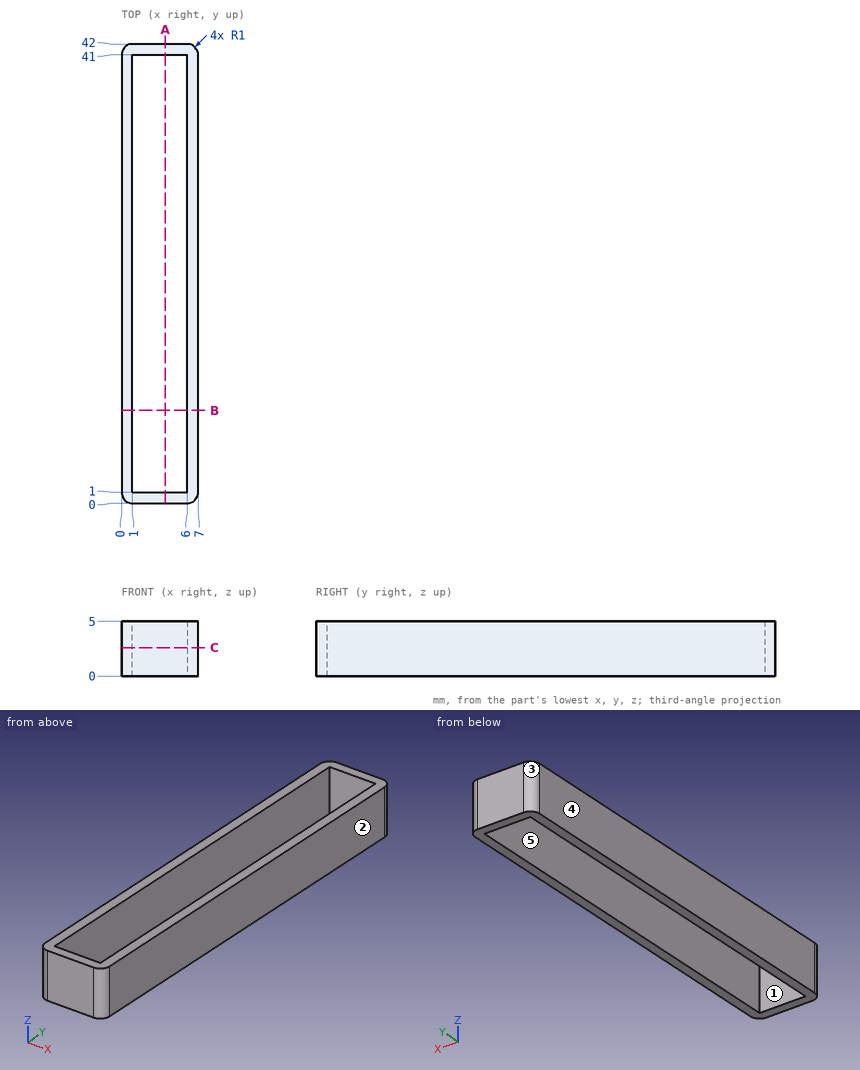
Could you check a few things on this drawing? It's one solid part, dimensions in mm from its lowest x, y, z. A direction names the side the tool comes from. Give positions to 0.01 mm unless a question says otherwise; leave off trailing zeros. Loops run counter-clockwise (first coordinate to the right, second up) from the corner with the lowest first, then second, coordinate; pieces in that order, holes last. Notation, with made-up numbers: M 68,63.5 L 84,63.5 A26 cw 84,84.5 Z; hole C 23.25,-18.75 d6. An arc over 180 degrees is marked long. Return JSON: item names as keys, results as strings.
Item 1: Imagine slicing it at C-C on z = 2.6. List the corners of the cut face in (x, y) for me, then the cut area to 3 significant figures.
A:
{"outline": "M 0,1 A1 ccw 1,0 L 6,0 A1 ccw 7,1 L 7,41 A1 ccw 6,42 L 1,42 A1 ccw 0,41 Z; hole M 1,1 L 6,1 L 6,41 L 1,41 Z", "area": "93.1 mm^2"}
Item 2: On a 3-axis mill with a long thin cutter (end or side, diameter ignored), from which of +Z, -Z, +X, -X, +Y, -Y can I reach the whole of each face in a straight line? I mean the marked faces 4 and 5. Say none if no direction works.
A:
{"face 4": "+Z, -Z, -X, +Y, -Y", "face 5": "+Z, -Z"}
Item 3: Please list where these lines run through material, in increasing order: line 1 (X direction, y = 20.5, z = 3.6); line 2 (Y direction, x = 4.25, z = 3.9).
A:
{"line 1": "x = 0 to 1, 6 to 7", "line 2": "y = 0 to 1, 41 to 42"}
Item 4: Imagine slicing it at B-B on y = 8.5. List the corners of the cut face in (x, z) for me, then the cut area to 3 significant figures.
A:
{"outline": "M 0,0 L 1,0 L 1,5 L 0,5 Z; M 6,0 L 7,0 L 7,5 L 6,5 Z", "area": "10.0 mm^2"}
Item 5: Imagine slicing it at A-A on x = 4. List the corners of the cut face in (y, z) for me, then the cut area to 3 significant figures.
A:
{"outline": "M 0,0 L 1,0 L 1,5 L 0,5 Z; M 41,0 L 42,0 L 42,5 L 41,5 Z", "area": "10.0 mm^2"}
Item 6: I'm going to push flat-ended pins straight in: pin 1 Ø1.5 at (x, y) = (5, 30.5) entering from +Z; pin 2 Ø1.5 at (x, y) = (1.5, 17) entering from -Z. Where does each tip first touch, or does it pass through?
A:
{"pin 1": "passes through", "pin 2": "stops at z = 0"}
Item 7: Thinking about a two-plate mould opening in Y: for the marked faces 1, 2 and 3, which applies, released by +Y, released by -Y, zero draft, split by the parting line, or undercut?
A:
{"face 1": "undercut", "face 2": "zero draft", "face 3": "released by +Y"}
